from build123d import *

# Parameters (mm, degrees)
SKETCH_3_R          = 2
CUT_EXTRUDE_4_DEPTH = 1
SKETCH_5_R          = 33.306153754
CUT_EXTRUDE_5_DEPTH = 1


with BuildPart() as part:
    # 草图1 → 旋转2 (revolve)
    with BuildSketch(Plane(origin=(0, 0, 0), x_dir=(0, 0, -1), z_dir=(1, 0, 0)), mode=Mode.PRIVATE) as revolve_2_sk:
        with BuildLine():
            Line((0, 0), (-23.5, 0))
            Line((-23.5, 0), (-23.5, 1))
            Line((-23.5, 1), (-13.5, 1))
            Line((-13.5, 1), (-13.5, 12))
            Line((-13.5, 12), (-5.196152423, 12))
            ThreePointArc((-5.196152423, 12), (-3, 14.196152423), (0, 15))
            Line((0, 15), (0, 9))
            Line((0, 9), (0, 0))
        make_face()
    revolve(revolve_2_sk.sketch.rotate(Axis((0, 0, 0), (0, 1, 0)), 180), axis=Axis((0, 0, 0), (0, 1, 0)))

    # 草图3 → 切除-拉伸4 (cut)
    with BuildSketch(Plane(origin=(0, 0, 0), x_dir=(1, 0, 0), z_dir=(0, 1, 0))):
        with Locations(Location((0, 17.5, 0), (0, 0, 90))):
            Circle(SKETCH_3_R)
        with Locations(Location((0, -17.5, 0), (0, 0, 90))):
            Circle(SKETCH_3_R)
    extrude(amount=CUT_EXTRUDE_4_DEPTH, mode=Mode.SUBTRACT)

    # 草图5 → 切除-拉伸5 (cut)
    with BuildSketch(Plane(origin=(0, 0, 0), x_dir=(1, 0, 0), z_dir=(0, 1, 0))):
        Circle(SKETCH_5_R)
        with BuildLine():
            Line((2.288026903, -22.440343498), (12.400353743, -10.516023969))
            ThreePointArc((12.400353743, -10.516023969), (16.259013902, 0), (12.400353743, 10.516023969))
            Line((12.400353743, 10.516023969), (2.288026903, 22.440343498))
            ThreePointArc((2.288026903, 22.440343498), (0, 23.5), (-2.288026903, 22.440343498))
            Line((-2.288026903, 22.440343498), (-12.400353743, 10.516023969))
            ThreePointArc((-12.400353743, 10.516023969), (-16.259013902, 0), (-12.400353743, -10.516023969))
            Line((-12.400353743, -10.516023969), (-2.288026903, -22.440343498))
            ThreePointArc((-2.288026903, -22.440343498), (0, -23.5), (2.288026903, -22.440343498))
        make_face(mode=Mode.SUBTRACT)
    extrude(amount=CUT_EXTRUDE_5_DEPTH, mode=Mode.SUBTRACT)


solid = part.part
Build history of the part. All positions in model axes, mm. A direction names the side the tool comes from. Give positions to 0.01 mm unless a question says otherwise; leave off trailing zeros. Loops run counter-clockwise (first coordinate to the right, second up) from the corner with the lowest first, then second, coordinate; pieces in that order, holes last. Notation, with made-up numbers: (81.25, 56.5) -> (135.25, 56.5) arc R17 cw to (135.25, 85.5) -> close; hole circle Ø10 at (-37.5, -4). An arc over 180 degrees is marked (long way). Answer in a Markdown table with one row per item.
Item 1: Slice it at B-B on x = 0. Write the cut outline in (y, z).
Findings below:
| item | result |
|---|---|
| outline | (0, -23.5) -> (1, -23.5) -> (1, -19.5) -> (0, -19.5) -> close; (0, -15.5) -> (1, -15.5) -> (1, -13.5) -> (12, -13.5) -> (12, -5.2) arc R6 ccw to (12, 5.2) -> (12, 13.5) -> (1, 13.5) -> (1, 15.5) -> (0, 15.5) -> close; (0, 19.5) -> (1, 19.5) -> (1, 23.5) -> (0, 23.5) -> close |
Item 2: Mould opens along X. For faces 3 (the flat face through (-7.273, 0.493, -16.562)), 4 (the cylindrical face through (1.2, 0.5, 19.1)), 5 (the cylindrical face through (16.26, 0.49, 0.16)), 6 (the cylindrical face through (1.2, 0.5, -15.9)) say: pulls with the +X half, pulls with the -X half, needs draft (parallel to the pull), parting line crosses it, or undercut.
Findings below:
| item | result |
|---|---|
| face 3 | pulls with the -X half |
| face 4 | undercut |
| face 5 | pulls with the +X half |
| face 6 | undercut |
Item 3: Slice it at D-D on z = 0. Write the cut outline in (x, y), plus the area to 3 significant figures.
Findings below:
| item | result |
|---|---|
| outline | (-16.26, 0) -> (16.26, 0) -> (16.26, 1) -> (13.5, 1) -> (13.5, 12) -> (5.2, 12) arc R6 ccw to (-5.2, 12) -> (-13.5, 12) -> (-13.5, 1) -> (-16.26, 1) -> close |
| area | 352 mm² |
Item 4: Flat gauge pins, fed straight in: P1, Ø1.5, axis at y = 8.5, z = 9, coming from the +X side; P2, Ø6, axis at x = -2, z = 9, coming from the -Y side; P3, Ø2.5, axis at x = 0, z = 17.5, coming from the -Y side; P4, Ø8, axis at y = 12.5, z = 11.5, coming from the -X side. Where does each tip first touch, or does it go through?
Findings below:
| item | result |
|---|---|
| P1 | stops at x = 10.69 |
| P2 | stops at y = 0 |
| P3 | passes through |
| P4 | stops at x = -11.2 |
Item 5: Slice it at C-C on y = 5.25. Write the cut outline in (x, z), plus the area to 3 significant figures.
Findings below:
| item | result |
|---|---|
| outline | circle Ø27 at (0, 0) |
| area | 573 mm² |
Item 6: Tool access for faces 1 (the cylindrical face through (13.18, 6.58, 2.93)), 2 (the cylindrical face through (-16.26, 0.49, -0.16)): list every direction of +Z, -Z, +X, -X, +Y, -Y with a clear straight run to the whole face (end or side of a thin tool).
Findings below:
| item | result |
|---|---|
| face 1 | +Y |
| face 2 | -X, +Y, -Y |
Item 7: Probe line 1 along Y through (x, z) = (8, 7); line 2 along X through (y, z) = (0.6, 17.5); line 3 along Y through (x, z) = (-15, 3). List the from-to ranges inside material, lowest first. Write a range as [from, to].
Findings below:
| item | result |
|---|---|
| line 1 | y = [0, 12] |
| line 2 | x = [-6.48, -2], [2, 6.48] |
| line 3 | y = [0, 1] |
Item 8: Slice it at A-A on z = -17.5. Write the cut outline in (x, y), plus the area to 3 significant figures.
Findings below:
| item | result |
|---|---|
| outline | (-6.48, 0) -> (-2, 0) -> (-2, 1) -> (-6.48, 1) -> close; (2, 0) -> (6.48, 0) -> (6.48, 1) -> (2, 1) -> close |
| area | 8.96 mm² |
